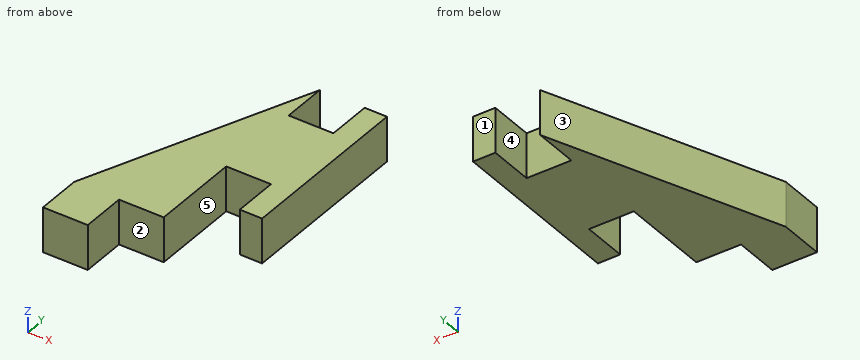
```python
from build123d import *

# Parameters (mm, degrees)
BOSS_EXTRUDE1_DEPTH = 6.35
SKETCH2_W           = 3.175
SKETCH2_H           = 25.4
BOSS_EXTRUDE2_DEPTH = 6.35


with BuildPart() as part:
    # Sketch1 → Boss-Extrude1 (new body)
    with BuildSketch(Plane.XY):
        Polygon((0, 0), (0, 12.7), (6.35, 12.7), (6.35, 25.4), (0, 25.4), (0, 31.75), (-12.7, 0), (-12.7, -6.35), (-6.35, -6.35), (-6.35, 0), align=None)
    extrude(amount=BOSS_EXTRUDE1_DEPTH)

    # Sketch2 → Boss-Extrude2 (add)
    with BuildSketch(Plane.XY):
        with Locations((7.9375, 19.05)):
            Rectangle(SKETCH2_W, SKETCH2_H)
    extrude(amount=BOSS_EXTRUDE2_DEPTH)


solid = part.part
```
Work out the finished part from the listing and answer in its coordinate system (mm). Face numbers are marked on the shaded views. A direction names the side the tool comes from. Coordinates: 2 decimals unless noted, no trailing zeros. Write each loop counter-clockwise with the first axis right and the second up, starting at its lowest first coordinate (ties: lowest second). Pieces come first, ordered by that corner, then holes.
Q1. A cutting plane is placed at C-C, the plane x = -4. Give the vertices of the cut face in (y, z), then the cut area to 3 significant figures.
Q2. A cutting plane is placed at D-D, the plane y = 17.5. Give the vertices of the cut face in (x, z) (3 decimals), then the cut area to 3 significant figures.
Q3. Which of the six approach directions +Z, -Z, +X, -X, +Y, -Y give full straight-line access (tool end or side, diameter ignored) to the marked faces 1, 2, 3, 4 and 5?
Q4. A cutting plane is placed at A-A, the plane y = 27.5. Give the vertices of the cut face in (x, z) (3 decimals), then the cut area to 3 significant figures.
Q5. Find the intervals of material crossed by line 1 (Y direction, x = 3.25, z = 0.5); line 2 (X direction, y = 29.5, z = 4.5) (3 decimals); line 3 (Y direction, x = 8, z = 2), in increasing order.
Q6. Each of these flat-tipped pins is pushed along its axis until it touches: pin 1 Ø1 at (x, z) = (7.5, 4.5) entering from -Y; pin 2 Ø1.9 at (x, z) = (2, 3.5) entering from +Y; pin 3 Ø1.9 at (y, z) = (4, 4.5) entering from +X. Where does it stop, or does it pass through?
Q7. A cutting plane is placed at B-B, the plane z = 1. Give the vertices of the cut face in (x, y) (3 decimals), then the cut area to 3 significant figures.
Findings below:
1. outline: (0, 0) - (21.75, 0) - (21.75, 6.35) - (0, 6.35) - close
1. area: 138 mm2
2. outline: (-5.7, 0) - (9.525, 0) - (9.525, 6.35) - (-5.7, 6.35) - close
2. area: 96.7 mm2
3. face 1: +Z, -Z, +X, -X, +Y
3. face 2: +Z, -Z, +X, -Y
3. face 3: +Z, -Z, -X, +Y
3. face 4: +Z, -Z, +Y
3. face 5: +Z, -Z, -Y
4. outline: (-1.7, 0) - (0, 0) - (0, 6.35) - (-1.7, 6.35) - close; (6.35, 0) - (9.525, 0) - (9.525, 6.35) - (6.35, 6.35) - close
4. area: 31.0 mm2
5. line 1: y = 12.7 to 25.4
5. line 2: x = -0.9 to 0, 6.35 to 9.525
5. line 3: y = 6.35 to 31.75
6. pin 1: stops at y = 6.35
6. pin 2: stops at y = 25.4
6. pin 3: stops at x = 0
7. outline: (-12.7, -6.35) - (-6.35, -6.35) - (-6.35, 0) - (0, 0) - (0, 12.7) - (6.35, 12.7) - (6.35, 6.35) - (9.525, 6.35) - (9.525, 31.75) - (6.35, 31.75) - (6.35, 25.4) - (0, 25.4) - (0, 31.75) - (-12.7, 0) - close
7. area: 403 mm2
